```python
from build123d import *

# Parameters (mm, degrees)
SKETCH2_W           = 30
SKETCH2_H           = 30
SKETCH2_W_2         = 20
SKETCH2_H_2         = 20
BOSS_EXTRUDE2_DEPTH = 3.5
SKETCH2_4_W         = 20
SKETCH2_4_H         = 20
BOSS_EXTRUDE3_DEPTH = 1
FILLET1_R           = 2
CUT_EXTRUDE1_DEPTH  = 4


with BuildPart() as part:
    # Sketch2 → Boss-Extrude2 (new body)
    with BuildSketch(Plane(origin=(0, 0, 0), x_dir=(1, 0, 0), z_dir=(0, 1, 0))):
        Rectangle(SKETCH2_W, SKETCH2_H)
        Rectangle(SKETCH2_W_2, SKETCH2_H_2, mode=Mode.SUBTRACT)
    extrude(amount=BOSS_EXTRUDE2_DEPTH)

    # Sketch2<4> → Boss-Extrude3 (add)
    with BuildSketch(Plane(origin=(0, 0, 0), x_dir=(1, 0, 0), z_dir=(0, 1, 0))):
        Rectangle(SKETCH2_4_W, SKETCH2_4_H)
    extrude(amount=BOSS_EXTRUDE3_DEPTH)

    # Fillet1
    fillet1_edges = [part.edges().sort_by_distance(p)[0] for p in [
        (-10, 1, 0),
        (0, 1, -10),
        (0, 1, 10),
        (10, 1, 0),
    ]]
    fillet(fillet1_edges, radius=FILLET1_R)

    # Sketch6 → Cut-Extrude1 (cut)
    with BuildSketch(Plane(origin=(0, 3.5, 0), x_dir=(1, 0, 0), z_dir=(0, 1, 0))):
        with BuildLine():
            ThreePointArc((-13.560660172, 13.560660172), (-13.560660172, 11.439339828), (-11.439339828, 11.439339828))
            Line((-11.439339828, 11.439339828), (-13.560660172, 13.560660172))
        make_face()
        with BuildLine():
            Line((-13.560660172, 13.560660172), (-11.439339828, 11.439339828))
            ThreePointArc((-11.439339828, 11.439339828), (-11.114180701, 11.925974851), (-11, 12.5))
            ThreePointArc((-11, 12.5), (-11.925974851, 13.885819299), (-13.560660172, 13.560660172))
        make_face()
        with BuildLine():
            ThreePointArc((13.560660172, 13.560660172), (11.439339828, 13.560660172), (11.439339828, 11.439339828))
            Line((11.439339828, 11.439339828), (13.560660172, 13.560660172))
        make_face()
        with BuildLine():
            Line((13.560660172, 13.560660172), (11.439339828, 11.439339828))
            ThreePointArc((11.439339828, 11.439339828), (13.074025149, 11.114180701), (14, 12.5))
            ThreePointArc((14, 12.5), (13.885819299, 13.074025149), (13.560660172, 13.560660172))
        make_face()
        with BuildLine():
            ThreePointArc((14, -12.5), (13.074025149, -11.114180701), (11.439339828, -11.439339828))
            Line((11.439339828, -11.439339828), (13.560660172, -13.560660172))
            ThreePointArc((13.560660172, -13.560660172), (13.885819299, -13.074025149), (14, -12.5))
        make_face()
        with BuildLine():
            Line((13.560660172, -13.560660172), (11.439339828, -11.439339828))
            ThreePointArc((11.439339828, -11.439339828), (11.439339828, -13.560660172), (13.560660172, -13.560660172))
        make_face()
        with BuildLine():
            ThreePointArc((-11, -12.5), (-11.114180701, -11.925974851), (-11.439339828, -11.439339828))
            Line((-11.439339828, -11.439339828), (-13.560660172, -13.560660172))
            ThreePointArc((-13.560660172, -13.560660172), (-11.925974851, -13.885819299), (-11, -12.5))
        make_face()
        with BuildLine():
            Line((-13.560660172, -13.560660172), (-11.439339828, -11.439339828))
            ThreePointArc((-11.439339828, -11.439339828), (-13.560660172, -11.439339828), (-13.560660172, -13.560660172))
        make_face()
    extrude(amount=-CUT_EXTRUDE1_DEPTH, mode=Mode.SUBTRACT)


solid = part.part
```
Work out the finished part from the listing and answer in its coordinate system (mm). A direction names the side the tool comes from. Give positions to 0.01 mm unless a question says otherwise; leave off trailing zeros. Loops run counter-clockwise (first coordinate to the right, second up) from the corner with the lowest first, then second, coordinate; pieces in that order, holes last. Notation, with made-up numbers: (9.25, 58.25) - (24.25, 58.25) arc R6 ccw to (24.25, 67.25) - close; hole circle Ø11 at (33, 73.25). An arc over 180 degrees is marked (long way). One line per question, with ' | ' between items.
(1) The mould has two halves that part along Z. Classify faces 3 (the face through (-15, 2, 0)), 4 (the face through (0, 2, 15)), 5 (the face through (9.43, 1.6, -0.14)): +Z half, -Z half, draft (parallel to the pull), parting line (faces both ways), or undercut.
Recorded:
face 3: draft | face 4: +Z half | face 5: undercut
(2) The part is cut by section B-B (z = 0). Write down the section's boundary in (x, y), then the cut area to 3 significant figures.
Recorded:
outline: (-15, 0) - (15, 0) - (15, 3.5) - (10, 3.5) - (10, 3) arc R2 cw to (8, 1) - (-8, 1) arc R2 cw to (-10, 3) - (-10, 3.5) - (-15, 3.5) - close | area: 56.7 mm²
(3) This flat-tipped pin is pushed along its axis until it touches: pin 1 Ø5 at (x, z) = (1.5, 2.5) entering from +Y. Where does it stop, or does it pass through?
Recorded:
pin 1: stops at y = 1
(4) The part is cut by section C-C (y = 2.15). Write down the section's boundary in (x, z).
Recorded:
outline: (-15, -15) - (15, -15) - (15, 15) - (-15, 15) - close; hole circle Ø3 at (-12.5, -12.5); hole circle Ø3 at (-12.5, 12.5); hole (-9.81, -9.81) - (9.81, -9.81) - (9.81, 9.81) - (-9.81, 9.81) - close; hole circle Ø3 at (12.5, -12.5); hole circle Ø3 at (12.5, 12.5)
(5) Straight lines are drawn through the part: probe 1 along Z at (x, y) = (13.5, 2.15); probe 2 along X at (y, z) = (2.65, -12.5); probe 3 along X at (y, z) = (1.5, -12). For each, find the intervals that lie inside material, in ascending order.
Recorded:
probe 1: z = -15 to -13.62, -11.38 to 11.38, 13.62 to 15 | probe 2: x = -15 to -14, -11 to 11, 14 to 15 | probe 3: x = -15 to -13.91, -11.09 to 11.09, 13.91 to 15
(6) The part is cut by section A-A (x = 12.75). Write down the section's boundary in (y, z).
Recorded:
outline: (0, -15) - (3.5, -15) - (3.5, -13.98) - (0, -13.98) - close; (0, -11.02) - (3.5, -11.02) - (3.5, 11.02) - (0, 11.02) - close; (0, 13.98) - (3.5, 13.98) - (3.5, 15) - (0, 15) - close
(7) A tool of negligible diameter and unlimited length cuts with its end or side. For faces 1 (the face through (0.14, 1.6, 9.43)), 2 (the face through (0, 0, 0)), from which of +Z, -Z, +X, -X, +Y, -Y can it reach the whole face along a straight path? Write none if from no direction.
Recorded:
face 1: +Y | face 2: +Z, -Z, +X, -X, -Y
(8) The part is cut by section D-D (x = -0.5). Write down the section's boundary in (y, z), then the cut area to 3 significant figures.
Recorded:
outline: (0, -15) - (3.5, -15) - (3.5, -10) - (3, -10) arc R2 cw to (1, -8) - (1, 8) arc R2 cw to (3, 10) - (3.5, 10) - (3.5, 15) - (0, 15) - close | area: 56.7 mm²
